Could you check a few things on this model? Use its own coordinates, in mm. Face numbers are marked on the shaded views. A direction names the side the tool comes from. Give positions to 0.01 mm unless a question says otherwise; leave off trailing zeros. Loops run counter-clockwise (first coordinate to the right, second up) from the corner with the lowest first, then second, coordinate; pieces in that order, holes last. Notation, with made-up numbers: M -35.5,61.5 L -4.5,61.5 A14 cw -4.5,76.5 Z; hole C 46,-19 d6. An arc over 180 degrees is marked long. Return JSON: item names as keys, results as strings. Group by question number.
1. Please list where these lines run through material, in increasing order: line 1 (Z direction, x = 9, y = -0.5); line 2 (Z direction, x = -6, y = 4.25); line 3 (Y direction, x = 1.5, z = 3.7).
2. If we section it at C-C (z = 2.7): Write out the boundary of the cut face in (x, y), plus the area to 3 significant figures.
3. For the marked faces 1 and 2, which set-ups out of +Z, -Z, +X, -X, +Y, -Y let a thin tool reach every point of the face, with its end or its side?
4. If we section it at D-D (z = 4.85): Write out the boundary of the cut face in (x, y).
5. For pin 1 (3 mm diameter, centred on x = 7, z = 1, fed in from -Y); pin 2 (5 mm diameter, centred on x = 4.5, y = -7, fed in from +Z); pin 3 (3 mm diameter, centred on x = -0.5, z = 3, fed in from +Y), each with a flat end and sliding along its axis, tell me the tip position at first contact or that it passes through.
```python
from build123d import *

# Parameters (mm, degrees)
F0_R     = 11
F0_R_2   = 7.5
F1_DEPTH = 2
F0_R_3   = 4.0165
F2_DEPTH = 3
F3_DEPTH = 5.5
F4_R     = 0.99999


# Not quite as in the source:
# - a fillet or chamfer is up to 0.001 mm smaller than in the source, because OpenCascade refuses the exact size


with BuildPart() as f1:
    # F0 (on Top) → F1 (new body)
    with BuildSketch(Plane.XY):
        Circle(F0_R)
        Circle(F0_R_2, mode=Mode.SUBTRACT)
    extrude(amount=F1_DEPTH)

    # F0 (on Top) → F2 (join)
    with BuildSketch(Plane.XY):
        Circle(F0_R_2)
        Circle(F0_R_3, mode=Mode.SUBTRACT)
    extrude(amount=F2_DEPTH)

    # F0 (on Top) → F3 (join)
    with BuildSketch(Plane.XY):
        Circle(F0_R_3)
    extrude(amount=F3_DEPTH)

    # F4 (radius 1 in the source; OpenCascade refuses exactly that, so slightly less here)
    f4_edges = [f1.edges().sort_by_distance(p)[0] for p in [
        (-11, 0, 2),
        (-11, 0, 0),
    ]]
    fillet(f4_edges, radius=F4_R)


solid = f1.part
```
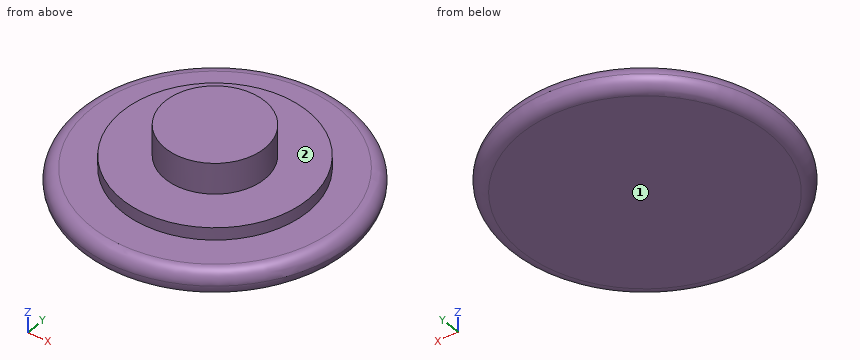
Answer:
{
 "1": {"line 1": "z = 0 to 2", "line 2": "z = 0 to 3", "line 3": "y = -3.73 to 3.73"},
 "2": {"outline": "C 0,0 d15", "area": "177 mm²"},
 "3": {"face 1": "-Z, +X, -X, +Y, -Y", "face 2": "+Z"},
 "4": {"outline": "C 0,0 d8.03"},
 "5": {"pin 1": "stops at y = -9.53", "pin 2": "stops at z = 3", "pin 3": "stops at y = 10.86"}
}
